```python
from build123d import *

# Parameters (mm, degrees)
F0_W     = 50
F0_H     = 40
F1_DEPTH = 50
F2_W     = 40
F2_H     = 40
F3_DEPTH = 50
F4_W     = 10
F4_H     = 30
F5_DEPTH = 10
F6_W     = 15
F6_H     = 10
F7_DEPTH = 10


with BuildPart() as f1:
    # F0 (on Front) → F1 (new body)
    with BuildSketch(Plane.XZ):
        with Locations((-60.347423, 20)):
            Rectangle(F0_W, F0_H)
    extrude(amount=F1_DEPTH)

    # F2 (on face) → F3 (cut)
    with BuildSketch(Plane.XY.offset(40)):
        with Locations((-65.347423, -20)):
            Rectangle(F2_W, F2_H)
    extrude(amount=-F3_DEPTH, mode=Mode.SUBTRACT)

    # F4 (on face) → F5 (cut)
    with BuildSketch(Plane.XZ.offset(50)):
        with Locations((-70.347423, 15)):
            Rectangle(F4_W, F4_H)
        with Locations((-50.347423, 15)):
            Rectangle(F4_W, F4_H)
    extrude(amount=-F5_DEPTH, mode=Mode.SUBTRACT)

    # F6 (on face) → F7 (cut)
    with BuildSketch(Plane.YZ.offset(-35.347423)):
        with Locations((-32.5, 25)):
            Rectangle(F6_W, F6_H)
        with Locations((-32.5, 5)):
            Rectangle(F6_W, F6_H)
    extrude(amount=-F7_DEPTH, mode=Mode.SUBTRACT)


solid = f1.part
```
Check sheet for the modelled part. Datum: model origin and axes. Units: mm. A direction names the side the tool comes from. Give positions to 0.01 mm unless a question says otherwise; leave off trailing zeros. Order: outer loops, then holes, each group sorted by start corner. A loop starts at its lowest first (then second) coordinate and runs counter-clockwise, first axis right, second up. Notation, with made-up numbers: M -13,77.25 L -2,77.25 A17 ccw -2,102.25 Z; hole C 15,34.25 d3. An arc over 180 degrees is marked long. Answer in a Markdown table with one row per item. Add a question column.
Q1. Access from +Z, -Z, +X, -X, +Y, -Y to the whole of each face (thin tool, end or side, straight path). Record for faces 5 (the flat face through (-40, -25, 5)), 6 (the flat face through (-40, -25, 25)), 7 (the flat face through (-61, -40, 25)).
Q2. Sectioned sample at D-D, the plane x = -42. Record the boundary of the cut face in (y, z).
Q3. Thickness scan on L1, parallel to Y at x = -39.5, z = 22.5; L2, parallel to X at y = -35, z = 34; L3, parallel to Y at x = -58, z = 33.5. Record the ranges inside material, lowest first.
Q4. Sectioned sample at A-A, the plane y = -37.5. Record the boundary of the cut face in (x, z).
Q5. Sectioned sample at B-B, the plane z = 14.5. Record the boundary of the cut face in (x, y), and give its area (3 significant figures).
Q6. Gauge pin test, flat ends, axial feed: pin 1 Ø12 at (x, z) = (-74, 6) entering from -Y; pin 2 Ø5 at (y, z) = (-29.5, 27) entering from -X; pin 3 Ø12 at (x, z) = (-57.5, 10.5) entering from +Y; pin 4 Ø5 at (x, y) = (-42.5, -29) entering from -Z. Record the tip position at first contact, or that the pin passes through.
Q7. Release check for a two-part mould opening along Z. For faces 1 (the flat face through (-85.347, -45, 20)), 2 (the flat face through (-40, -40, 25)), 3 (the flat face through (-40, -33, 30)), 4 (the flat face through (-60, -45, 0)) record: released by +Z, released by -Z, zero draft, split by the parting line, or undercut.
Q8. Sectioned sample at C-C, the plane z = 7. Record the boundary of the cut face in (x, y), and give its area (3 significant figures).
Verdict:
| question | item | result |
|---|---|---|
| 1 | face 5 | -Z, +X, -X |
| 1 | face 6 | +X, -X |
| 1 | face 7 | +Z, -Z, -X, +Y |
| 2 | outline | M -50,0 L -40,0 L -40,10 L -25,10 L -25,0 L 0,0 L 0,40 L -50,40 Z; hole M -40,20 L -25,20 L -25,30 L -40,30 Z |
| 3 | L1 | -50 to -40, -25 to 0 |
| 3 | L2 | -45.35 to -35.35 |
| 3 | L3 | -50 to -40 |
| 4 | outline | M -45.35,10 L -35.35,10 L -35.35,20 L -45.35,20 Z; M -45.35,30 L -35.35,30 L -35.35,40 L -45.35,40 Z |
| 5 | outline | M -85.35,-50 L -75.35,-50 L -75.35,-40 L -85.35,-40 Z; M -65.35,-50 L -55.35,-50 L -55.35,-40 L -65.35,-40 Z; M -45.35,-50 L -35.35,-50 L -35.35,0 L -45.35,0 Z |
| 5 | area | 700 mm² |
| 6 | pin 1 | y = -50 |
| 6 | pin 2 | through |
| 6 | pin 3 | y = -40 |
| 6 | pin 4 | z = 10 |
| 7 | face 1 | zero draft |
| 7 | face 2 | undercut |
| 7 | face 3 | undercut |
| 7 | face 4 | released by -Z |
| 8 | outline | M -85.35,-50 L -75.35,-50 L -75.35,-40 L -85.35,-40 Z; M -65.35,-50 L -55.35,-50 L -55.35,-40 L -65.35,-40 Z; M -45.35,-50 L -35.35,-50 L -35.35,-40 L -45.35,-40 Z; M -45.35,-25 L -35.35,-25 L -35.35,0 L -45.35,0 Z |
| 8 | area | 550 mm² |
